```python
from build123d import *

# Parameters (mm, degrees)
F0_W         = 108.5126549006
F0_H         = 71.473672986
F0_R         = 19.6812167499
F0_W_2       = 29.5154461637
F0_H_2       = 21.7025321908
F0_R_2       = 5.5283506547
F0_R_3       = 6.3923279955
F1_DEPTH     = 25.4
F2_T1_DEPTH  = 29.5154461637
F2_T3_DEPTH  = 133.9126549006
F2_T5_DEPTH  = 96.873672986
F2_T7_DEPTH  = 21.7025321908
F2_T19_DEPTH = 34.4025321908
F2_T23_DEPTH = 42.2154461637
F2_T30_DEPTH = 42.2154461637
F2_T34_DEPTH = 34.4025321908
F2_T41_DEPTH = 34.4025321908
F2_T45_DEPTH = 42.2154461637
F2_T52_DEPTH = 34.4025321908
F2_T56_DEPTH = 42.2154461637


# Not quite as in the source:
# - a fillet or chamfer that OpenCascade refuses, or shapes differently, is made with other operations: its cross-section is extruded or revolved along the edge and cut away or added


with BuildPart() as f1:
    # F0 (on Right) → F1 (new body)
    with BuildSketch(Plane.YZ):
        with Locations((-1.3021528721, -0.2893656492)):
            Rectangle(F0_W, F0_H)
        with Locations((-26.6217719764, -9.1150635853)):
            Circle(F0_R, mode=Mode.SUBTRACT)
        with Locations((26.6217733733, -13.0215191748)):
            Rectangle(F0_W_2, F0_H_2, mode=Mode.SUBTRACT)
        with Locations((-38.775190711, 22.1365820616)):
            Circle(F0_R_2, mode=Mode.SUBTRACT)
        with Locations((35.01342237, 25.3196209669)):
            Circle(F0_R_3, mode=Mode.SUBTRACT)
    extrude(amount=F1_DEPTH)

    # F2: fillet of radius 5.08 on 11 edges, made by hand

    # F2_s2 → F2_t1 (cut)
    with BuildSketch(Plane.XZ.offset(-41.3794964552)):
        with BuildLine():
            ThreePointArc((20.32, -2.1702530794), (23.9121024484, -0.6823555278), (25.4, 2.9097469206))
            Line((25.4, 2.9097469206), (25.4, -2.1702530794))
            Line((25.4, -2.1702530794), (20.32, -2.1702530794))
        make_face()
        with BuildLine():
            ThreePointArc((20.32, -23.8727852702), (23.9121024484, -25.3606828218), (25.4, -28.9527852702))
            Line((25.4, -28.9527852702), (25.4, -23.8727852702))
            Line((25.4, -23.8727852702), (20.32, -23.8727852702))
        make_face()
    extrude(amount=F2_T1_DEPTH, mode=Mode.SUBTRACT)

    # F2_s4 → F2_t3 (cut)
    with BuildSketch(Plane.XZ.offset(-65.6541745782)):
        with BuildLine():
            ThreePointArc((20.32, 35.4474708438), (23.9121024484, 33.9595732922), (25.4, 30.3674708438))
            Line((25.4, 30.3674708438), (25.4, 35.4474708438))
            Line((25.4, 35.4474708438), (20.32, 35.4474708438))
        make_face()
        with BuildLine():
            ThreePointArc((20.32, -36.0262021422), (23.9121024484, -34.5383045907), (25.4, -30.9462021422))
            Line((25.4, -30.9462021422), (25.4, -36.0262021422))
            Line((25.4, -36.0262021422), (20.32, -36.0262021422))
        make_face()
    extrude(amount=F2_T3_DEPTH, mode=Mode.SUBTRACT)

    # F2_s6 → F2_t5 (cut)
    with BuildSketch(Plane.XY.offset(-48.7262021422)):
        with BuildLine():
            ThreePointArc((20.32, -55.5584803224), (23.9121024484, -54.0705827708), (25.4, -50.4784803224))
            Line((25.4, -50.4784803224), (25.4, -55.5584803224))
            Line((25.4, -55.5584803224), (20.32, -55.5584803224))
        make_face()
        with BuildLine():
            ThreePointArc((20.32, 52.9541745782), (23.9121024484, 51.4662770266), (25.4, 47.8741745782))
            Line((25.4, 47.8741745782), (25.4, 52.9541745782))
            Line((25.4, 52.9541745782), (20.32, 52.9541745782))
        make_face()
    extrude(amount=F2_T5_DEPTH, mode=Mode.SUBTRACT)

    # F2_s8 → F2_t7 (cut)
    with BuildSketch(Plane.XY.offset(-23.8727852702)):
        with BuildLine():
            ThreePointArc((20.32, 11.8640502915), (23.9121024484, 10.3761527399), (25.4, 6.7840502915))
            Line((25.4, 6.7840502915), (25.4, 11.8640502915))
            Line((25.4, 11.8640502915), (20.32, 11.8640502915))
        make_face()
        with BuildLine():
            ThreePointArc((20.32, 41.3794964552), (23.9121024484, 42.8673940068), (25.4, 46.4594964552))
            Line((25.4, 46.4594964552), (25.4, 41.3794964552))
            Line((25.4, 41.3794964552), (20.32, 41.3794964552))
        make_face()
    extrude(amount=F2_T7_DEPTH, mode=Mode.SUBTRACT)

    # F2_s9 → F2_t10 (revolve, cut)
    with BuildSketch(Plane.XY.offset(-9.1150635853)):
        with BuildLine():
            ThreePointArc((20.32, -6.9405552264), (23.9121024484, -5.4526576749), (25.4, -1.8605552264))
            Line((25.4, -1.8605552264), (25.4, -6.9405552264))
            Line((25.4, -6.9405552264), (20.32, -6.9405552264))
        make_face()
    revolve(axis=Axis((25.4, -26.6217719764, -9.1150635853), (1, 0, 0)), mode=Mode.SUBTRACT)

    # F2_s11 → F2_t12 (revolve, cut)
    with BuildSketch(Plane.XY.offset(22.1365820616)):
        with BuildLine():
            ThreePointArc((20.32, -33.2468400563), (23.9121024484, -31.7589425047), (25.4, -28.1668400563))
            Line((25.4, -28.1668400563), (25.4, -33.2468400563))
            Line((25.4, -33.2468400563), (20.32, -33.2468400563))
        make_face()
    revolve(axis=Axis((25.4, -38.775190711, 22.1365820616), (1, 0, 0)), mode=Mode.SUBTRACT)

    # F2_s13 → F2_t14 (revolve, cut)
    with BuildSketch(Plane.XY.offset(25.3196209669)):
        with BuildLine():
            ThreePointArc((20.32, 41.4057503654), (23.9121024484, 42.893647917), (25.4, 46.4857503654))
            Line((25.4, 46.4857503654), (25.4, 41.4057503654))
            Line((25.4, 41.4057503654), (20.32, 41.4057503654))
        make_face()
    revolve(axis=Axis((25.4, 35.01342237, 25.3196209669), (1, 0, 0)), mode=Mode.SUBTRACT)


with BuildPart() as f2_tool17:
    # F2_s18 → F2_t19 (new body)
    with BuildSketch(Plane.XY.offset(-23.8727852702)):
        with BuildLine():
            ThreePointArc((20.32, 11.8640502915), (23.9121024484, 10.3761527399), (25.4, 6.7840502915))
            Line((25.4, 6.7840502915), (25.4, 11.8640502915))
            Line((25.4, 11.8640502915), (20.32, 11.8640502915))
        make_face()
    extrude(amount=F2_T19_DEPTH)

    split(bisect_by=Plane.XY.offset(-2.1702530794), keep=Keep.TOP)


with BuildPart() as f2_tool21:
    # F2_s22 → F2_t23 (new body)
    with BuildSketch(Plane.XZ.offset(0.8359497085)):
        with BuildLine():
            ThreePointArc((20.32, -2.1702530794), (23.9121024484, -0.6823555278), (25.4, 2.9097469206))
            Line((25.4, 2.9097469206), (25.4, -2.1702530794))
            Line((25.4, -2.1702530794), (20.32, -2.1702530794))
        make_face()
    extrude(amount=-F2_T23_DEPTH)

    split(bisect_by=Plane.XZ.offset(-11.8640502915), keep=Keep.TOP)


with BuildPart() as f2_tool17_1:
    add(f2_tool17.part)

    # F2_t25: intersect F2_tool21
    add(f2_tool21.part, mode=Mode.INTERSECT)


with BuildPart() as f1_1:
    add(f1.part)

    # F2_t15: cut F2_tool17
    add(f2_tool17_1.part, mode=Mode.SUBTRACT)


with BuildPart() as f2_tool28:
    # F2_s29 → F2_t30 (new body)
    with BuildSketch(Plane.XZ.offset(-11.8640502915)):
        with BuildLine():
            ThreePointArc((20.32, -2.1702530794), (23.9121024484, -0.6823555278), (25.4, 2.9097469206))
            Line((25.4, 2.9097469206), (25.4, -2.1702530794))
            Line((25.4, -2.1702530794), (20.32, -2.1702530794))
        make_face()
    extrude(amount=-F2_T30_DEPTH)

    split(bisect_by=Plane.XZ.offset(-41.3794964552), keep=Keep.BOTTOM)


with BuildPart() as f2_tool32:
    # F2_s33 → F2_t34 (new body)
    with BuildSketch(Plane.XY.offset(10.5297469206)):
        with BuildLine():
            ThreePointArc((20.32, 41.3794964552), (23.9121024484, 42.8673940068), (25.4, 46.4594964552))
            Line((25.4, 46.4594964552), (25.4, 41.3794964552))
            Line((25.4, 41.3794964552), (20.32, 41.3794964552))
        make_face()
    extrude(amount=-F2_T34_DEPTH)

    split(bisect_by=Plane.XY.offset(-2.1702530794), keep=Keep.TOP)


with BuildPart() as f2_tool28_1:
    add(f2_tool28.part)

    # F2_t36: intersect F2_tool32
    add(f2_tool32.part, mode=Mode.INTERSECT)


with BuildPart() as f1_2:
    add(f1_1.part)

    # F2_t26: cut F2_tool28
    add(f2_tool28_1.part, mode=Mode.SUBTRACT)


with BuildPart() as f2_tool39:
    # F2_s40 → F2_t41 (new body)
    with BuildSketch(Plane.XY.offset(-36.5727852702)):
        with BuildLine():
            ThreePointArc((20.32, 11.8640502915), (23.9121024484, 10.3761527399), (25.4, 6.7840502915))
            Line((25.4, 6.7840502915), (25.4, 11.8640502915))
            Line((25.4, 11.8640502915), (20.32, 11.8640502915))
        make_face()
    extrude(amount=F2_T41_DEPTH)

    split(bisect_by=Plane.XY.offset(-23.8727852702), keep=Keep.BOTTOM)


with BuildPart() as f2_tool43:
    # F2_s44 → F2_t45 (new body)
    with BuildSketch(Plane.XZ.offset(-41.3794964552)):
        with BuildLine():
            ThreePointArc((20.32, -23.8727852702), (23.9121024484, -25.3606828218), (25.4, -28.9527852702))
            Line((25.4, -28.9527852702), (25.4, -23.8727852702))
            Line((25.4, -23.8727852702), (20.32, -23.8727852702))
        make_face()
    extrude(amount=F2_T45_DEPTH)

    split(bisect_by=Plane.XZ.offset(-11.8640502915), keep=Keep.TOP)


with BuildPart() as f2_tool39_1:
    add(f2_tool39.part)

    # F2_t47: intersect F2_tool43
    add(f2_tool43.part, mode=Mode.INTERSECT)


with BuildPart() as f1_3:
    add(f1_2.part)

    # F2_t37: cut F2_tool39
    add(f2_tool39_1.part, mode=Mode.SUBTRACT)


with BuildPart() as f2_tool50:
    # F2_s51 → F2_t52 (new body)
    with BuildSketch(Plane.XY.offset(-2.1702530794)):
        with BuildLine():
            ThreePointArc((20.32, 41.3794964552), (23.9121024484, 42.8673940068), (25.4, 46.4594964552))
            Line((25.4, 46.4594964552), (25.4, 41.3794964552))
            Line((25.4, 41.3794964552), (20.32, 41.3794964552))
        make_face()
    extrude(amount=-F2_T52_DEPTH)

    split(bisect_by=Plane.XY.offset(-23.8727852702), keep=Keep.BOTTOM)


with BuildPart() as f2_tool54:
    # F2_s55 → F2_t56 (new body)
    with BuildSketch(Plane.XZ.offset(-54.0794964552)):
        with BuildLine():
            ThreePointArc((20.32, -23.8727852702), (23.9121024484, -25.3606828218), (25.4, -28.9527852702))
            Line((25.4, -28.9527852702), (25.4, -23.8727852702))
            Line((25.4, -23.8727852702), (20.32, -23.8727852702))
        make_face()
    extrude(amount=F2_T56_DEPTH)

    split(bisect_by=Plane.XZ.offset(-41.3794964552), keep=Keep.BOTTOM)


with BuildPart() as f2_tool50_1:
    add(f2_tool50.part)

    # F2_t58: intersect F2_tool54
    add(f2_tool54.part, mode=Mode.INTERSECT)


with BuildPart() as f1_4:
    add(f1_3.part)

    # F2_t48: cut F2_tool50
    add(f2_tool50_1.part, mode=Mode.SUBTRACT)


solid = f1_4.part
```
Read the model definition and answer for the solid it produces. Units are mm, in the model's axes. A direction names the side the tool comes from. Give positions to 0.01 mm unless a question says otherwise; leave off trailing zeros. Write each loop counter-clockwise with the first axis right and the second up, starting at its lowest first coordinate (ties: lowest second). Pieces come first, ordered by that corner, then holes. Notation, with made-up numbers: (14, 10) - (27, 10) arc R17 cw to (27, 24) - close; hole circle Ø3 at (-21, 82). An arc over 180 degrees is marked (long way). Write item = value, one per line. Start each with the question number.
Item 1: Find section A-A (y = 19.5). Give the vertices of the cut face in (x, z), then the cut area to 3 significant figures.
Item 2: Find section C-C (y = 30.5). State how many separate pieces and enclosed holes the cut face has, then the cut area to 3 significant figures.
Item 3: Each of these flat-tipped pins is pushed along its axis until it touches: P1, Ø20.5, axis at y = 35.01, z = 25.32, coming from the +X side; P2, Ø3, axis at x = 22, y = 23, coming from the -Z side. Where does it stop, or does it pass through?
Item 4: Find the intervals of material crossed by probe 1 along Y at (x, z) = (2.25, 26); probe 2 along Z at (x, y) = (4.75, -38); probe 3 along Z at (x, y) = (20, 27), in increasing order. Write a range as [from, to].
Item 5: The mould has two halves that part along Y. Classify faces 1 (the flat face through (10, -55.558, -1)), 2 (the cylindrical face through (23.87, 10.42, -13.24)), 3 (the flat face through (25.4, 7, 14)): +Y half, -Y half, draft (parallel to the pull), parting line (faces both ways), or undercut.
Item 6: A tool of negligible diameter and unlimited length cuts with its end or side. For faces 4 (the flat face through (25.4, -48, 14)), 5 (the flat face through (10, 26, -23.873)), 6 (the cylindrical face through (23.872, 42.828, -13.245)), from which of +Z, -Z, +X, -X, +Y, -Y can it reach the whole face along a straight path? Write none if from no direction.
Item 7: Find section B-B (x = 16.5). Give the vertices of the cut face in (y, z), then the cut area to 3 significant figures.
Response:
q1.outline = (0, -36.03) - (20.32, -36.03) arc R5.08 ccw to (25.4, -30.95) - (25.4, -28.95) arc R5.08 ccw to (20.32, -23.87) - (0, -23.87) - close; (0, -2.17) - (20.32, -2.17) arc R5.08 ccw to (25.4, 2.91) - (25.4, 30.37) arc R5.08 ccw to (20.32, 35.45) - (0, 35.45) - close
q1.area = 1,240 mm²
q2.separate_pieces = 3
q2.enclosed_holes = 0
q2.area = 999 mm²
q3.P1 = 25.25
q3.P2 = -36.02
q4.probe_1 = [-55.56, -42.73], [-34.82, 28.66], [41.37, 52.95]
q4.probe_2 = [-36.03, -25.17], [6.94, 16.66], [27.61, 35.45]
q4.probe_3 = [-36.03, -23.87], [-2.17, 35.45]
q5.face_1 = -Y half
q5.face_2 = undercut
q5.face_3 = draft
q6.face_4 = +Z, -Z, +X, +Y, -Y
q6.face_5 = +X, -X
q6.face_6 = +X
q7.outline = (-55.56, -36.03) - (52.95, -36.03) - (52.95, 35.45) - (-55.56, 35.45) - close; hole circle Ø39.36 at (-26.62, -9.12); hole circle Ø11.06 at (-38.78, 22.14); hole (11.86, -23.87) - (41.38, -23.87) - (41.38, -2.17) - (11.86, -2.17) - close; hole circle Ø12.78 at (35.01, 25.32)
q7.area = 5,670 mm²
